Check sheet for the modelled part. Datum: model origin and axes. Units: mm. A direction names the side the tool comes from. Give positions to 0.01 mm unless a question says otherwise; leave off trailing zeros. Order: outer loops, then holes, each group sorted by start corner. A loop starts at its lowest first (then second) coordinate and runs counter-clockwise, first axis right, second up.
from build123d import *

# Parameters (mm, degrees)
SKETCH1_R           = 1.5
BOSS_EXTRUDE1_DEPTH = 4.7625
SKETCH2_R           = 2.15265
CUT_EXTRUDE1_DEPTH  = 61.429350536
SKETCH3_W           = 19.05
SKETCH3_H           = 19.05
CUT_EXTRUDE2_DEPTH  = 3.699999966


with BuildPart() as part:
    # Sketch1 → Boss-Extrude1 (new, symmetric)
    with BuildSketch(Plane(origin=(0, 0, 0), x_dir=(1, 0, 0), z_dir=(0, 1, 0))):
        Polygon((-14.9225, -4.1275), (-14.9225, -9.525), (57.15, -9.525), (57.15, 9.525), (20.0025, 9.525), (20.0025, 4.1275), (4.1275, 4.1275), (4.1275, -4.1275), align=None)
        with Locations(Location((50.8, 0, 0), (0, 0, 90))):
            Circle(SKETCH1_R, mode=Mode.SUBTRACT)
    extrude(amount=BOSS_EXTRUDE1_DEPTH, both=True)

    # Sketch2 → Cut-Extrude1 (cut, through all)
    with BuildSketch(Plane.XY.offset(9.525)):
        with Locations((-9.525, 0)):
            Circle(SKETCH2_R)
        with Locations((11.1125, 0)):
            Circle(SKETCH2_R)
    extrude(amount=-CUT_EXTRUDE1_DEPTH, mode=Mode.SUBTRACT)

    # Sketch3 → Cut-Extrude2 (cut)
    with BuildSketch(Plane.XZ.offset(4.7625)):
        with Locations((47.625, 0)):
            Rectangle(SKETCH3_W, SKETCH3_H)
    extrude(amount=-CUT_EXTRUDE2_DEPTH, mode=Mode.SUBTRACT)


solid = part.part
1) Set-up check for faces 4 (the face through (20.002, 0, -7)), 5 (the face through (47, -1.063, 0)), 6 (the face through (39, 1, -9.525)): record each of +Z, -Z, +X, -X, +Y, -Y from which the full face is reachable in a straight line by a thin tool's end or side.
Recorded:
face 4: -Z, -X, +Y, -Y
face 5: +Z, -Z, +X, -Y
face 6: -Z, +X, -X, +Y, -Y
2) Depth check by flat-ended pin: pin 1 Ø4 at (y, z) = (-1.5, 0) entering from -X; pin 2 Ø1.5 at (y, z) = (-2.5, 5.5) entering from +X; pin 3 Ø1.8 at (x, z) = (50.8, 0) entering from +Y; pin 4 Ø5.5 at (x, z) = (52, -0.5) entering from -Y. Enter the tip coordinate at first touch or a pass-through.
Recorded:
pin 1: stops at x = 4.13
pin 2: stops at x = 38.1
pin 3: passes through
pin 4: stops at y = -1.06
3) Draft check along Y on faces 1 (the face through (38.1, -3, 0)), 2 (the face through (8.96, 0.09, 2.79)), 3 (the face through (17, -4.762, 2)). Enter one of: +Y half, -Y half, draft (parallel to the pull), parting line (faces both ways), or undercut.
Recorded:
face 1: draft
face 2: undercut
face 3: -Y half
4) Section check C-C, the plane y = 0. State how many separate pieces and enclosed holes the cut face has, then the cut area to 3 significant figures.
Recorded:
separate pieces: 3
enclosed holes: 1
area: 938 mm2
5) Material ranges on L1, parallel to X at y = 2.2, z = 0; L2, parallel to X at y = 1.3, z = 0; L3, parallel to Z at x = 50.8, y = 1.1 (3 decimals), recorded low to high.
Recorded:
L1: x = 4.13 to 49.3, 52.3 to 57.15
L2: x = 4.13 to 9.4, 12.83 to 49.3, 52.3 to 57.15
L3: z = -9.525 to -1.5, 1.5 to 9.525
6) Section check A-A, the plane z = 0. Record the cut outline in (x, y), then the cut area to 3 significant figures.
Recorded:
outline: (4.13, -4.76) - (38.1, -4.76) - (38.1, -1.06) - (49.3, -1.06) - (49.3, 4.76) - (4.13, 4.76) - close; (52.3, -1.06) - (57.15, -1.06) - (57.15, 4.76) - (52.3, 4.76) - close; hole circle Ø4.31 at (11.11, 0)
area: 403 mm2
7) Section check B-B, the plane x = 50.8. Record the cut outline in (y, z) (1 decimal), then the cut area to 3 significant figures.
Recorded:
outline: (-1.1, -9.5) - (4.8, -9.5) - (4.8, -1.5) - (-1.1, -1.5) - close; (-1.1, 1.5) - (4.8, 1.5) - (4.8, 9.5) - (-1.1, 9.5) - close
area: 93.5 mm2
